Read the model definition and answer for the solid it produces. Units are mm, in the model's axes. A direction names the side the tool comes from. Coordinates: 2 decimals unless noted, no trailing zeros. Order: outer loops, then holes, each group sorted by start corner. A loop starts at its lowest first (then second) coordinate and runs counter-clockwise, first axis right, second up. Notation, with made-up numbers: M 6.5,53 L 65.5,53 A23 cw 65.5,82 Z; hole C 66,67 d4. An arc over 180 degrees is marked long. One line per question, with ' | ' between items. Start each with the question number.
1) Find section D-D, the plane x = -35. Write down the section's boundary in (y, z), plus the area to 3 significant figures.
2) A tool of negligible diameter and unlimited length cuts with its end or side. For faces 1 (the face through (-91.185, 20.327, 15.301)), 2 (the face through (-95, 2, 12)), 3 (the face through (-88, 23, 42)), 4 (the face through (-65, 0, 1)), from which of +Z, -Z, +X, -X, +Y, -Y can it reach the whole face along a straight path? Write none if from no direction.
3) Given P1, Ø9, axis at x = -95, z = 13, coming from the -Y side; P2, Ø2.5, axis at x = -95, z = 14.1, coming from the -Y side; P3, Ø21, axis at y = 30.5, z = 43.5, coming from the -X side, each flat-ended and moving along its own axis, determine where each tip first touches the part or whether it passes through.
4) Consider probe 1 along X at (y, z) = (9, 14); probe 2 along Z at (x, y) = (-67, 20); probe 3 along X at (y, z) = (19, 19). Determine where each line is inside the solid, lowest interval first.
5) Find section A-A, the plane y = 17.5. Write down the section's boundary in (x, z).
6) The mould has two halves that part along Z. Classify faces 5 (the face through (0, 23, 42)), 6 (the face through (-54, 23, 85)), 7 (the face through (-95, 17, 27.5)): +Z half, -Z half, draft (parallel to the pull), parting line (faces both ways), or undercut.
7) Find section C-C, the plane z = 33.5. Write down the section's boundary in (x, y), plus the area to 3 significant figures.
from build123d import *

# Parameters (mm, degrees)
SALIENTE_EXTRUIR1_DEPTH = 85
CROQUIS3_W              = 18
CROQUIS3_H              = 26
CORTAR_EXTRUIR1_DEPTH   = 47
VACIADO1_T              = -2
SALIENTE_EXTRUIR2_REACH = 48
CROQUIS4_R              = 4
CROQUIS5_R              = 4
CORTAR_EXTRUIR2_DEPTH   = 2
CROQUIS8_W              = 2
CROQUIS8_H              = 81
CORTAR_EXTRUIR3_DEPTH   = 2
CROQUIS9_R              = 1.5
CORTAR_EXTRUIR4_DEPTH   = 10


with BuildPart() as part:
    # Croquis2 → Saliente-Extruir1 (new body)
    with BuildSketch(Plane.XY):
        Polygon((0, 0), (0, 46), (-88, 46), (-106, 24), (-106, 0), align=None)
    extrude(amount=SALIENTE_EXTRUIR1_DEPTH)

    # Croquis3 → Cortar-Extruir1 (cut, through all)
    with BuildSketch(Plane.XZ):
        with Locations((-97, 42.5)):
            Rectangle(CROQUIS3_W, CROQUIS3_H)
    extrude(amount=-CORTAR_EXTRUIR1_DEPTH, mode=Mode.SUBTRACT)

    # Vaciado1
    vaciado1_openings = [part.faces().sort_by_distance(p)[0] for p in [
        (-75, 0, 42.5),
    ]]
    offset(amount=VACIADO1_T, openings=vaciado1_openings, kind=Kind.INTERSECTION)

    # Croquis4 → Saliente-Extruir2 (add, up to next)
    with BuildSketch(Plane.XZ, mode=Mode.PRIVATE) as saliente_extruir2_sk1:
        with Locations((-95, 69.6)):
            Circle(CROQUIS4_R)
    saliente_extruir2_tool1 = extrude(saliente_extruir2_sk1.sketch, amount=-SALIENTE_EXTRUIR2_REACH, mode=Mode.PRIVATE) - part.part
    add(saliente_extruir2_tool1.solids().sort_by_distance((-95, 0, 69.6))[0])
    # Croquis4 → Saliente-Extruir2 (add, up to next)
    with BuildSketch(Plane.XZ, mode=Mode.PRIVATE) as saliente_extruir2_sk2:
        with Locations((-95, 14.1)):
            Circle(CROQUIS4_R)
    saliente_extruir2_tool2 = extrude(saliente_extruir2_sk2.sketch, amount=-SALIENTE_EXTRUIR2_REACH, mode=Mode.PRIVATE) - part.part
    add(saliente_extruir2_tool2.solids().sort_by_distance((-95, 0, 14.1))[0])

    # Croquis5 → Cortar-Extruir2 (cut)
    with BuildSketch(Plane.XZ):
        with Locations((-95, 69.6)):
            Circle(CROQUIS5_R)
        with Locations((-95, 14.1)):
            Circle(CROQUIS5_R)
    extrude(amount=-CORTAR_EXTRUIR2_DEPTH, mode=Mode.SUBTRACT)

    # Croquis8 → Cortar-Extruir3 (cut)
    with BuildSketch(Plane.XZ):
        with Locations((-1, 42.5)):
            Rectangle(CROQUIS8_W, CROQUIS8_H)
    extrude(amount=-CORTAR_EXTRUIR3_DEPTH, mode=Mode.SUBTRACT)

    # Croquis9 → Cortar-Extruir4 (cut)
    with BuildSketch(Plane.XZ.offset(-2)):
        with Locations((-95, 69.6)):
            Circle(CROQUIS9_R)
        with Locations((-95, 14.1)):
            Circle(CROQUIS9_R)
    extrude(amount=-CORTAR_EXTRUIR4_DEPTH, mode=Mode.SUBTRACT)


solid = part.part
Report:
1) outline: M 0,0 L 46,0 L 46,85 L 0,85 L 0,83 L 44,83 L 44,2 L 0,2 Z | area: 346 mm^2
2) face 1: -Y | face 2: +X, -Y | face 3: -X, +Y, -Y | face 4: +Z, -Z, +X, -X, -Y
3) P1: stops at y = 2 | P2: stops at y = 12 | P3: stops at x = -88
4) probe 1: x = -106 to -104, -99 to -96.5, -93.5 to -91, -2 to 0 | probe 2: z = 0 to 2, 83 to 85 | probe 3: x = -106 to -104, -2 to 0
5) outline: M -106,0 L 0,0 L 0,85 L -106,85 L -106,55.5 L -88,55.5 L -88,29.5 L -106,29.5 Z; C -95,14.1 d8; C -95,69.6 d8; hole M -104,2 L -2,2 L -2,83 L -104,83 L -104,57.5 L -86,57.5 L -86,27.5 L -104,27.5 Z
6) face 5: draft | face 6: +Z half | face 7: undercut
7) outline: M -88,0 L -86,0 L -86,44 L -2,44 L -2,2 L 0,2 L 0,46 L -88,46 Z | area: 348 mm^2
